from build123d import *

# Parameters (mm, degrees)
TORUS_R           = 1
TORUS_ANGLE       = 90
CYLINDER002_R     = 1
CYLINDER002_DEPTH = 30
CYLINDER004_R     = 1
CYLINDER004_DEPTH = 48


with BuildPart() as torus:
    # Torus → Torus (revolve)
    with BuildSketch(Plane(origin=(24, 120, 0), x_dir=(1, 0, 0), z_dir=(0, -1, 0))):
        with Locations((4, 0)):
            Circle(TORUS_R)
    revolve(axis=Axis((24, 120, 0), (0, 0, 1)), revolution_arc=TORUS_ANGLE)


with BuildPart() as collector002:
    # Cylinder002 → Cylinder002 (new body)
    with BuildSketch(Plane(origin=(-28, 120, 0), x_dir=(1, 0, 0), z_dir=(0, -1, 0))):
        Circle(CYLINDER002_R)
    extrude(amount=CYLINDER002_DEPTH)


with BuildPart() as obj1:
    # Part__Mirroring002: instance of Collector002
    add(collector002.part.mirror(Plane(origin=(0, 0, 0), x_dir=(0, -1, 0), z_dir=(1, 0, 0))))


with BuildPart() as cylinder:
    # Cylinder004 → Cylinder004 (new body)
    with BuildSketch(Plane(origin=(-24, 124, 0), x_dir=(0, 0, -1), z_dir=(1, 0, 0))):
        Circle(CYLINDER004_R)
    extrude(amount=CYLINDER004_DEPTH)


with BuildPart() as obj2:
    # Part__Mirroring003: instance of Torus
    add(torus.part.mirror(Plane(origin=(0, 0, 0), x_dir=(0, -1, 0), z_dir=(1, 0, 0))))

    # Fusion: union Torus, Collector002, obj1, Cylinder
    add(torus.part)
    add(collector002.part)
    add(obj1.part)
    add(cylinder.part)


with BuildPart() as obj2_1:
    # Fusion placement: moved
    add(obj2.part.moved(Location((0, 0, -20))))


solid = obj2_1.part
Could you check a few things on this model? Use its own coordinates, in mm. A direction names the side the tool comes from. Give positions to 0.01 mm unless a question says otherwise; leave off trailing zeros. Order: outer loops, then holes, each group sorted by start corner. A loop starts at its lowest first (then second) coordinate and runs counter-clockwise, first axis right, second up.
1. Which directions (+Z, -Z, +X, -X, +Y, -Y) give clear straight access to the entire face, cutting with the end or side of a thin tool? Please do faces 3 (the cylindrical face through (-28, 105, -21)), 4 (the cylindrical face through (0, 123, -20)), 5 (the flat face through (-28, 90, -20)).
Answers below:
face 3: -Y
face 4: none
face 5: +Z, -Z, +X, -X, -Y
2. Thinking about a two-plate mould opening in X: for faces 1 (the flat face through (28, 90, -20)), 2 (the cylindrical face through (28, 105, -21)), which applies, +X half, -X half, draft (parallel to the pull), parting line (faces both ways), or undercut?
Answers below:
face 1: draft
face 2: undercut
3. Suppose I cut it at A-A (z = -20). Write out the boundary of the cut face in (x, y).
Answers below:
outline: (-29, 90) - (-27, 90) - (-27, 120) arc R3 cw to (-24, 123) - (24, 123) arc R3 cw to (27, 120) - (27, 90) - (29, 90) - (29, 120) arc R5 ccw to (24, 125) - (-24, 125) arc R5 ccw to (-29, 120) - close
4. Suppose I cut it at C-C (x = -15). Write out the boundary of the cut face in (y, z), plus the area to 3 significant figures.
Answers below:
outline: circle Ø2 at (124, -20)
area: 3.14 mm2
5. For pin 1 (6 mm diameter, centred on x = 5, y = 118, fed in from +Z), with a flat end and sliding along its axis, tell me the tip position at first contact or that it passes through.
Answers below:
pin 1: passes through
6. Suppose I cut it at B-B (y = 103.5). Write out the boundary of the cut face in (x, z).
Answers below:
outline: circle Ø2 at (-28, -20); circle Ø2 at (28, -20)
7. I need wall thicknesses on L1, parallel to X at y = 107, z = -19.85; L2, parallel to Y at x = -21.5, z = -20.15; L3, parallel to X at y = 106, z = -20.85. Which ranges of each line are inside material? Lowest first, please.
Answers below:
L1: x = -28.99 to -27.01, 27.01 to 28.99
L2: y = 123.01 to 124.99
L3: x = -28.53 to -27.47, 27.47 to 28.53
